Autodesk Fusion 360 part; units mm, degrees
sketch "草图1" plane through (0, 0, 0) normal (0, 0, 1) x (1, 0, 0)
  line L0 (10.0747, -14.9164) -> (21.7546, -35.3287)
  line L1 (15.0116, -9.9324) -> (35.2699, -21.7355)
  arc A0 (46.7824, -17.6466) -> (17.6321, -46.7879) centre (0, 0) ccw
  arc A1 (15.0116, -9.9324) -> (10.0747, -14.9164) centre (0, 0) ccw
  arc A2 (17.6321, -46.7879) -> (21.7546, -35.3287) centre (14.8109, -39.3019) ccw
  arc A3 (35.2699, -21.7355) -> (46.7824, -17.6466) centre (39.2972, -14.8232) ccw
  dimension "d1" = 100
  dimension "d2" = 36
  dimension "d3" = 8
extrude "拉伸1" add sketch "草图1" along normal blind 50
fillet "圆角1" radius 5 5 edges at (25.1407, -15.8339, 50) (41.9747, -22.3618, 50) (-35.3498, 35.3608, 50) (22.3386, -42.01, 50) (15.9146, -25.1226, 50)
fillet "圆角2" radius 5 5 edges at (10.0747, -14.9164, 22.5) (8.8197, -15.6912, 48.5451) (-12.7906, 12.6649, 50) (15.7752, -8.6685, 48.5475) (15.0116, -9.9324, 22.5)
fillet "圆角3" radius 5 8 edges at (17.0957, -27.1866, 0) (9.791, -16.8234, 0) (-12.7654, 12.6903, 0) (16.8692, -9.6593, 0) (27.1639, -17.0127, 0) (41.9747, -22.3618, 0) (-35.3498, 35.3608, 0) (22.3386, -42.01, 0)
Design review of the part built by this model. Coordinates are the model's own, in mm. A direction names the side the tool comes from. Round coordinates to 2 decimals unless told otherwise and drop trailing zeros. Loops run counter-clockwise (first coordinate to the right, second up) from the corner with the lowest first, then second, coordinate; pieces in that order, holes last. Notation, with made-up numbers: M 67,47.5 L 107,47.5 A18 ccw 107,71.5 Z; hole C 17.25,60 d10. An arc over 180 degrees is marked long. Answer as a JSON object with one key per item and string values.
Item 1: Wall thickness on L1, parallel to X at y = -13.5, z = 26; L2, parallel to X at y = -3.5, z = 25; L3, parallel to Y at x = -11, z = 3: over which ranges is each line inside the solid? List them lowest first. Write a range as from..to.
Answer sheet:
{"L1": "x = -48.14..-11.91, 21.13..48.14", "L2": "x = -49.88..-17.66, 17.66..49.88", "L3": "y = -48.35..-14.77, 14.77..48.35"}
Item 2: We need section A-A on z = 7. Give the boundary of the cut face in (x, y), and give its area (3 significant figures).
Answer sheet:
{"outline": "M 6.34,-16.85 A18 cw long 16.88,-6.24 A5 ccw 19.06,-12.29 L 35.27,-21.74 A8 ccw 46.78,-17.65 A50 ccw long 17.63,-46.79 A8 ccw 21.75,-35.33 L 12.44,-19.04 A5 ccw Z", "area": "6,300 mm^2"}
Item 3: The part is to be moulded in two halves that separate along X. For faces 1 (the flat face through (27.05, -16.947, 24.72)), 2 (the flat face through (-21, 11, 50)), 3 (the cylindrical face through (-36.67, 33.99, 24.72)), say which applies: pulls with the +X half, pulls with the -X half, needs draft (parallel to the pull), parting line crosses it, or undercut.
Answer sheet:
{"face 1": "undercut", "face 2": "needs draft", "face 3": "parting line crosses it"}
Item 4: Clearance check with flat-ended pins moving along their axes: P1, Ø21.5, axis at x = 0, y = 0, coming from the -Z side; P2, Ø3, axis at x = -30.5, z = 18, coming from the -Y side; P3, Ø10, axis at y = 8, z = 43.5, coming from the -X side; P4, Ø6, axis at x = 25, z = 20.5, coming from the -Y side. State where each tip first meets the part, or that it passes through.
Answer sheet:
{"P1": "passes through", "P2": "stops at y = -40.73", "P3": "stops at x = -49.91", "P4": "stops at y = -42.81"}
Item 5: Machinability: for faces 4 (the cylindrical face through (9.84, -16.84, 25.28)), 5 (the cylindrical face through (42.066, -22.329, 24.72)), which of the approach directions +Z, -Z, +X, -X, +Y, -Y give a long, thin tool a straight path to every point of the face, cutting with its end or side? Answer none if there is none.
Answer sheet:
{"face 4": "+Z, -Z", "face 5": "+Z, -Z, -Y"}
